The model under review builds one solid part; all positions refer to its coordinate system, in mm. Face numbers are marked on the shaded views. A direction names the side the tool comes from. Round coordinates to 2 decimals unless told otherwise and drop trailing zeros. Loops run counter-clockwise (first coordinate to the right, second up) from the corner with the lowest first, then second, coordinate; pieces in that order, holes last. Notation, with made-up numbers: M -7.5,43 L 20.5,43 A23 ccw 20.5,70 Z; hole C -29,66.25 d2. An arc over 180 degrees is marked long. Use a Markdown table: item, result. Add a question column.
```python
from build123d import *

# Parameters (mm, degrees)
BOSS_EXTRUDE1_DEPTH   = 13.6
M5X0_8_TAPPED_HOLE1_D = 4.2


with BuildPart() as part:
    # Sketch1 → Boss-Extrude1 (new body)
    with BuildSketch(Plane.XY):
        with BuildLine():
            Line((2.8, 0), (-2.8, 0))
            Line((-2.8, 0), (-2.8, -0.5))
            Line((-2.8, -0.5), (-4.15, -0.5))
            Line((-4.15, -0.5), (-4.15, -1.3))
            ThreePointArc((-4.15, -1.3), (-3.300609665, -3.350609665), (-1.25, -4.2))
            Line((-1.25, -4.2), (1.25, -4.2))
            ThreePointArc((1.25, -4.2), (3.300609665, -3.350609665), (4.15, -1.3))
            Line((4.15, -1.3), (4.15, -0.5))
            Line((4.15, -0.5), (2.8, -0.5))
            Line((2.8, -0.5), (2.8, 0))
        make_face()
    extrude(amount=BOSS_EXTRUDE1_DEPTH)

    # M5x0.8 Tapped Hole1 (through all)
    with Locations(Plane(origin=(0, 0, 0), x_dir=(1, 0, 0), z_dir=(0, 1, 0))):
        with Locations((0, -4.2)):
            Hole(M5X0_8_TAPPED_HOLE1_D / 2)


solid = part.part
```
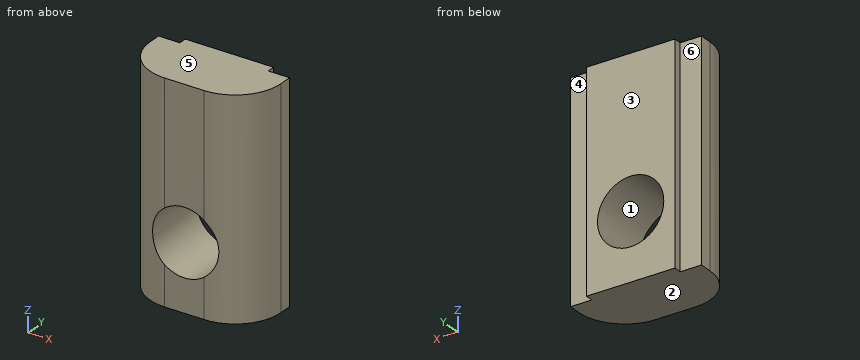
(1) To check wall thickness, follow probe 1 along Z at (x, y) = (-1.25, -4); probe 2 along Z at (x, y) = (0, -3.15); probe 3 along X at (y, z) = (-1.45, 10.25). State the ranges of each line that lie inside material, in increasing order.
(2) Insertion check: pin 1 Ø0.7 at (x, z) = (-3.5, 5.5) entering from +Y. The pin has a flat end and moves straight along its axis. Give the tip position at first contact, or say it passes through.
(3) Consider section C-C, the plane y = -0.75. Give the boundary of the cut face in (x, z), then the cut area to 3 significant figures.
(4) Consider section A-A, the plane x = 0. Give the boundary of the cut face in (y, z), then the cut area to 3 significant figures.
(5) Consider section B-B, the plane z = 4.2. Give the boundary of the cut face in (x, y).
(6) For the marked faces 4, 5 and 6, list the 3-axis set-ups (+Z, -Z, +X, -X, +Y, -Y) from which the entire face can be reached by the end or side of a thin tool; tool diameter is ignored.
(7) Draft analysis for pull direction Z (two halves, no side actions). For the marked faces 1, 2 and 3, state which applies: released by +Z, released by -Z, zero draft, split by the parting line, or undercut.
(8) Consider section D-D, the plane z = 9.75. Give the boundary of the cut face in (x, y).
Found:
| question | item | result |
|---|---|---|
| 1 | probe 1 | z = 0 to 2.51, 5.89 to 13.6 |
| 1 | probe 2 | z = 0 to 2.1, 6.3 to 13.6 |
| 1 | probe 3 | x = -4.15 to 4.15 |
| 2 | pin 1 | stops at y = -0.5 |
| 3 | outline | M -4.15,0 L 4.15,0 L 4.15,13.6 L -4.15,13.6 Z; hole C 0,4.2 d4.2 |
| 3 | area | 99.0 mm^2 |
| 4 | outline | M -4.2,0 L 0,0 L 0,2.1 L -4.2,2.1 Z; M -4.2,6.3 L 0,6.3 L 0,13.6 L -4.2,13.6 Z |
| 4 | area | 39.5 mm^2 |
| 5 | outline | M -4.15,-1.3 A2.9 ccw -2.1,-4.07 L -2.1,0 L -2.8,0 L -2.8,-0.5 L -4.15,-0.5 Z; M 2.1,-4.07 A2.9 ccw 4.15,-1.3 L 4.15,-0.5 L 2.8,-0.5 L 2.8,0 L 2.1,0 Z |
| 6 | face 4 | +Z, -Z, +X, +Y |
| 6 | face 5 | +Z, +X, -X, +Y, -Y |
| 6 | face 6 | +Z, -Z, -X, +Y |
| 7 | face 1 | undercut |
| 7 | face 2 | released by -Z |
| 7 | face 3 | zero draft |
| 8 | outline | M -4.15,-1.3 A2.9 ccw -1.25,-4.2 L 1.25,-4.2 A2.9 ccw 4.15,-1.3 L 4.15,-0.5 L 2.8,-0.5 L 2.8,0 L -2.8,0 L -2.8,-0.5 L -4.15,-0.5 Z |
